Geometry: final body of the model. Coordinates: model frame, mm. Face numbers are marked on the shaded views. A direction names the side the tool comes from. Coordinates: 2 decimals unless noted, no trailing zeros. Loops run counter-clockwise (first coordinate to the right, second up) from the corner with the lowest first, then second, coordinate; pieces in that order, holes last. Notation, with made-up numbers: (-23, 53.5) - (24, 53.5) arc R34 ccw to (24, 92.5) - close; hole circle Ø6 at (-29, 4.25). An arc over 180 degrees is marked (long way). Answer in a Markdown table with one row per item.
Autodesk Fusion 360 part; units mm, degrees
sketch "Sketch2" plane through (0, 0, 0) normal (0, 0, 1) x (1, 0, 0)
  line L0 (0, 0) -> (40, 0)
  line L1 (40, 0) -> (40, 71)
  line L2 (40, 71) -> (0, 71)
  line L3 (0, 71) -> (0, 0)
  line L4 (2, 2) -> (38, 2)
  line L5 (38, 2) -> (38, 69)
  line L6 (38, 69) -> (2, 69)
  line L7 (2, 69) -> (2, 2)
  dimension "d1" = 40
  dimension "d2" = 71
  dimension "d26" = 67
extrude "Extrude1" add sketch "Sketch2" along normal blind 9.4
sketch "Sketch3" plane through (0, 0, 0) normal (0, 0, 1) x (1, 0, 0)
  line L0 (2, 2) -> (38, 2)
  line L1 (38, 2) -> (38, 69.0002)
  line L2 (38, 69.0002) -> (2, 69.0002)
  line L3 (2, 69.0002) -> (2, 2)
extrude "Extrude2" add sketch "Sketch3" along normal blind 1.4
sketch "Sketch4" plane through (0, 0, 1.4) normal (0, 0, 1) x (-1, 0, 0)
  line L0 (-2, -69) -> (-2, -2)
  line L1 (-2, -2) -> (-38, -2)
  line L2 (-38, -2) -> (-38, -69)
  line L3 (-25, -30) -> (-15, -30)
  line L4 (-15, -30) -> (-15, -40)
  line L5 (-15, -40) -> (-25, -40)
  line L6 (-25, -40) -> (-25, -30)
  line L7 (-38, -69) -> (-2, -69)
extrude "Extrude3" add sketch "Sketch4" along normal blind 3 contours L3 L4 L5 L6
extrude "Extrude4" add 1 faces at (21.6667, 33.3333, 4.4) along direction (0, 0, 1) blind 1.5
hole "Hole1" at (20, 71, 5.9) direction (0, -1, 0) diameter 5.5 depth 74 tip angle 118
hole "Hole2" at (31.1767, 2, 6.3948) direction (0, -1, 0) diameter 8.3 depth 10 tip angle 118
sketch "Sketch5" plane through (0, 40, 0) normal (0, 1, 0) x (-1, 0, 0)
  arc A0 (-22.75, 5.9) -> (-17.25, 5.9) centre (-20, 5.9) ccw
  line L0 (-22.75, 5.9) -> (-25, 5.9)
  line L1 (-25, 5.9) -> (-25, 1.4)
  line L2 (-25, 1.4) -> (-15, 1.4)
  line L3 (-15, 1.4) -> (-15, 5.9)
  line L4 (-15, 5.9) -> (-17.25, 5.9)
sketch "Sketch6" plane through (0, 40, 0) normal (0, 1, 0) x (-1, 0, 0)
  line L0 (-25, 1.4) -> (-21.5733, 1.4)
  line L1 (-21.5733, 1.4) -> (-21.5733, 3.205)
  line L2 (-21.5733, 3.205) -> (-23.2867, 3.205)
  line L3 (-25, 3.205) -> (-25, 1.4)
  line L4 (-23.2867, 3.205) -> (-25, 4)
  line L5 (-25, 4) -> (-25, 3.205)
extrude "Extrude5" cut sketch "Sketch6" against normal blind 8.5
extrude "Extrude6" add 1 faces at (24.1592, 30, 4.0023) along direction (0, -1, 0) blind 8
sketch "Sketch7" plane through (0, 0, 9.4) normal (0, 0, 1) x (-1, 0, 0)
  line L0 (-28.3147, 0) -> (-28.3147, -2)
  line L1 (-28.3147, -2) -> (-2, -2)
  line L2 (-2, -2) -> (-2, -69)
  line L3 (-2, -69) -> (-38, -69)
  line L4 (-38, -69) -> (-38, -2)
  line L5 (-38, -2) -> (-34.0387, -2)
  line L6 (-34.0387, -2) -> (-34.0387, 0)
  line L7 (-34.0387, 0) -> (-40, 0)
  line L8 (-40, 0) -> (-40, -71)
  line L9 (-40, -71) -> (0, -71)
  line L10 (0, -71) -> (0, 0)
  line L11 (0, 0) -> (-28.3147, 0)
  line L12 (-40, -69) -> (-24.0637, -69)
  line L13 (-24.0637, -69) -> (-24.0637, -71)
  line L14 (-24.0637, -71) -> (-40, -71)
  line L15 (-40, -71) -> (-40, -69)
extrude "Extrude7" cut sketch "Sketch7" against normal blind 8 contours L3 L8 L9 L12 L13 L14 L15
sketch "Sketch8" plane through (0, 0, 9.4) normal (0, 0, 1) x (-1, 0, 0)
  line L0 (-40, -69) -> (-38, -69)
  line L1 (-38, -69) -> (-38, -2)
  line L2 (-38, -2) -> (-34.0387, -2)
  line L3 (-34.0387, -2) -> (-34.0387, 0)
  line L4 (-34.0387, 0) -> (-40, 0)
  line L5 (-40, 0) -> (-40, -69)
  line L6 (-40, -69) -> (-38, -69)
  line L7 (-38, -69) -> (-38, -62)
  line L8 (-38, -62) -> (-40, -62)
  line L9 (-40, -62) -> (-40, -69)
extrude "Extrude8" cut sketch "Sketch8" against normal blind 8 contours L0 L1 L5 L6 L7 L8 L9
extrude "Extrude9" add 1 faces at (24.1592, 22, 4.0023) along direction (0, -1, 0) blind 6
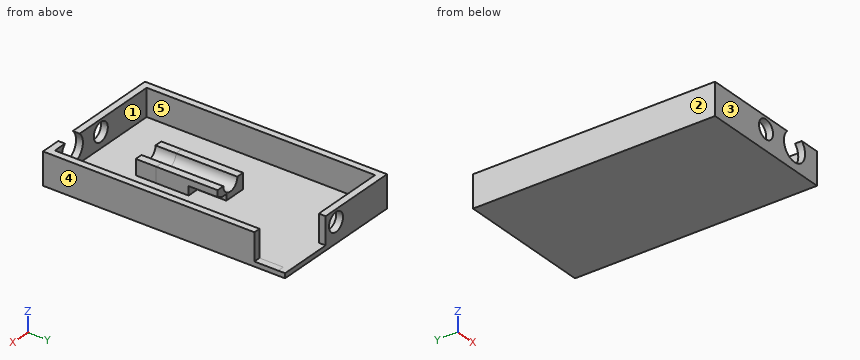
(1) Cut plane D-D on x = 5.5. Output: boundary loops of the cut face in (y, z).
Verdict:
| item | result |
|---|---|
| outline | (0, 0) - (71, 0) - (71, 9.4) - (69, 9.4) - (69, 1.4) - (2, 1.4) - (2, 9.4) - (0, 9.4) - close |
(2) Pull-direction query (Y, two-part tool) for the marked faces 3, 4 and 5; classes: pulls with the +Y half, pulls with the -Y half, needs draft (parallel to the pull), parting line crosses it, or undercut.
Verdict:
| item | result |
|---|---|
| face 3 | pulls with the -Y half |
| face 4 | needs draft |
| face 5 | undercut |
(3) Ray query, probe 1 along Y at (x, z) = (24, 1.75); probe 2 along Y at (x, z) = (21.5, 3.5); probe 3 along X at (y, z) = (24.5, 2.25). Return the intervals inside material, ascending.
Verdict:
| item | result |
|---|---|
| probe 1 | y = 0 to 2, 16 to 31.5, 69 to 71 |
| probe 2 | y = 0 to 2, 16 to 40, 69 to 71 |
| probe 3 | x = 0 to 2, 15 to 25, 38 to 40 |
(4) Cut plane B-B on y = 42. Output: boundary loops of the cut face in (x, z).
Verdict:
| item | result |
|---|---|
| outline | (0, 0) - (40, 0) - (40, 9.4) - (38, 9.4) - (38, 1.4) - (2, 1.4) - (2, 9.4) - (0, 9.4) - close |
(5) Cut plane A-A on x = 20. Output: boundary loops of the cut face in (y, z).
Verdict:
| item | result |
|---|---|
| outline | (0, 0) - (71, 0) - (71, 3.15) - (69, 3.15) - (69, 1.4) - (40, 1.4) - (40, 3.15) - (16, 3.15) - (16, 1.4) - (2, 1.4) - (2, 3.15) - (0, 3.15) - close; (0, 8.65) - (2, 8.65) - (2, 9.4) - (0, 9.4) - close; (69, 8.65) - (71, 8.65) - (71, 9.4) - (69, 9.4) - close |
(6) Cut plane C-C on z = 7.5. Output: boundary loops of the cut face in (x, y).
Verdict:
| item | result |
|---|---|
| outline | (0, 0) - (17.76, 0) - (17.76, 2) - (2, 2) - (2, 69) - (17.76, 69) - (17.76, 71) - (0, 71) - close; (22.24, 0) - (27.18, 0) - (27.18, 2) - (22.24, 2) - close; (22.24, 69) - (24.06, 69) - (24.06, 71) - (22.24, 71) - close; (35.18, 0) - (40, 0) - (40, 62) - (38, 62) - (38, 2) - (35.18, 2) - close |
(7) First-contact query: pin 1 Ø6 at (x, y) = (33, 22.5) entering from +Z; pin 2 Ø5 at (x, y) = (13.5, 17) entering from -Z; pin 3 Ø3.5 at (x, z) = (20, 5.9) entering from +Y; pin 4 Ø0.7 at (x, y) = (24, 20) entering from +Z. Flat tips, straight axial feed; report the tip coordinate or a pass-through.
Verdict:
| item | result |
|---|---|
| pin 1 | stops at z = 1.4 |
| pin 2 | stops at z = 0 |
| pin 3 | passes through |
| pin 4 | stops at z = 5.9 |
(8) Access query for the marked faces 1 and 2. Directions: +Z, -Z, +X, -X, +Y, -Y. A direction counts if a zero-diameter tool reaches every point of the face in a straight line with its end or side. Return the directions, or none.
Verdict:
| item | result |
|---|---|
| face 1 | +Z |
| face 2 | +Z, -Z, -X, +Y, -Y |
